Here's how the part is built. I have some questions about the finished solid (model axes, mm). A direction names the side the tool comes from. Round coordinates to 2 decimals unless told otherwise and drop trailing zeros. Loops run counter-clockwise (first coordinate to the right, second up) from the corner with the lowest first, then second, coordinate; pieces in that order, holes last. Notation, with made-up numbers: M 14.25,66 L 47.25,66 A15 ccw 47.25,80 Z; hole C 53.25,45 d6. An arc over 180 degrees is marked long. Use a Markdown table: item, result.
```python
from build123d import *

# Parameters (mm, degrees)
SKETCH2_R           = 19.05
SKETCH3_W           = 101.6
SKETCH3_H           = 101.6
BOSS_EXTRUDE1_DEPTH = 38.1


with BuildPart() as part:
    # Sweep1: sweep along a path in Sketch1
    with BuildLine(Plane(origin=(0, 0, 0), x_dir=(1, 0, 0), z_dir=(0, 1, 0))) as sweep1_path:
        Line((57.15, 0), (19.05, 0))
        ThreePointArc((19.05, 0), (5.579615818, 5.579615818), (0, 19.05))
        Line((0, 19.05), (0, 57.15))
    # Sketch2 → Sweep1 (sweep)
    with BuildSketch(Plane(origin=(57.15, 0, 0), x_dir=(0, 0, -1), z_dir=(1, 0, 0))):
        Circle(SKETCH2_R)
    sweep(path=sweep1_path.line)

    # Sketch3 → Boss-Extrude1 (add)
    with BuildSketch(Plane(origin=(0, 0, -57.15), x_dir=(-1, 0, 0), z_dir=(0, 0, -1))):
        Rectangle(SKETCH3_W, SKETCH3_H)
    extrude(amount=BOSS_EXTRUDE1_DEPTH)


solid = part.part
```
Q1. Will these pins go through, and if not, where does the flat tip stop? P1, Ø12, axis at y = 11.5, z = -7.5, coming from the -X side; P2, Ø19, axis at y = 2, z = -78.5, coming from the +X side.
Return value:
| item | result |
|---|---|
| P1 | stops at x = -16.98 |
| P2 | stops at x = 50.8 |
Q2. Imagine slicing it at A-A, the plane z = -42. Please give me the cut outline in (x, y).
Return value:
| item | result |
|---|---|
| outline | C 0,0 d38.1 |
Q3. For faces 1 (the cylindrical face through (10.241, -16.063, -38.367)), 2 (the flat face through (50.8, -1, -76)), 3 (the flat face through (57.15, 0, 0)), which set-ups out of +Z, -Z, +X, -X, +Y, -Y let a thin tool reach every point of the face, with its end or its side?
Return value:
| item | result |
|---|---|
| face 1 | none |
| face 2 | -Z, +X, +Y, -Y |
| face 3 | +Z, -Z, +X, +Y, -Y |
Q4. We'd pull the mould along Z, two halves only. Please class faces 4 (the flat face through (1, 1, -95.25)), 5 (the cylindrical face through (37.83, 11.59, 15.12)), 6 (the flat face through (1, -50.8, -76)): pulls with the +Z half, pulls with the -Z half, needs draft (parallel to the pull), parting line crosses it, or undercut.
Return value:
| item | result |
|---|---|
| face 4 | pulls with the -Z half |
| face 5 | undercut |
| face 6 | needs draft |
Q5. I need wall thicknesses on line 1 (Y direction, x = 0.5, z = -57); line 2 (X direction, y = 38.5, z = -90); line 3 (Z direction, x = 31.5, y = 26.5). Which ranges of each line are inside material? Lowest first, please. Write a range as from..to.
Return value:
| item | result |
|---|---|
| line 1 | y = -19.04..19.04 |
| line 2 | x = -50.8..50.8 |
| line 3 | z = -95.25..-57.15 |
Q6. Imagine slicing it at B-B, the plane y = 33. Please give me the cut outline in (x, z).
Return value:
| item | result |
|---|---|
| outline | M -50.8,-95.25 L 50.8,-95.25 L 50.8,-57.15 L -50.8,-57.15 Z |
